Check sheet for the modelled part. Datum: model origin and axes. Units: mm. A direction names the side the tool comes from. Round coordinates to 2 decimals unless told otherwise and drop trailing zeros. Order: outer loops, then holes, each group sorted by start corner. A loop starts at its lowest first (then second) coordinate and runs counter-clockwise, first axis right, second up.
Q1. Set-up check for faces 1 (the cylindrical face through (17.15, 2.46, -19.99)), 2 (the flat face through (50, 3.48, -6.03)): record each of +Z, -Z, +X, -X, +Y, -Y from which the full face is reachable in a straight line by a thin tool's end or side.
Q2. Cross-section at D-D on x = 33. Record the cut outline in (y, z).
Q3. Depth check by flat-ended pin: P1, Ø5, axis at x = 5, z = 28, coming from the -Y side; P2, Ø12, axis at x = 39.31, z = -8.69, coming from the +Y side; P3, Ø2, axis at y = 1.5, z = 25.5, coming from the -X side; P4, Ø1, axis at x = -43, y = 3.5, coming from the -Z side. Enter the tip coordinate at first touch or a pass-through.
Q4. Cross-section at A-A on x = -5. Record the cut outline in (y, z), then the cut area to 3 significant figures.
Q5. Cross-section at C-C on y = 3.5. Give the number of separate pieces and of enclosed holes in the cut face, then the cut area to 3 significant figures.
Q6. Scan lines: probe 1 along X at (y, z) = (2.75, -28); probe 2 along Z at (x, y) = (17.5, 3.6); probe 3 along Z at (x, y) = (-8.5, 4.5). Record each from-to range of solid material in increasing order.
Q7. Cross-section at B-B on z = 28. Record the cut outline in (x, y).
from build123d import *

# Parameters (mm, degrees)
CROQUIS1_R              = 1.6
CROQUIS1_R_2            = 4.6875
SALIENTE_EXTRUIR1_DEPTH = 5
CORTAR_EXTRUIR1_START   = -3
CROQUIS2_R              = 3
CROQUIS2_R_2            = 1.6
CROQUIS2_R_3            = 4.6875
CORTAR_EXTRUIR1_DEPTH   = 3


with BuildPart() as part:
    # Croquis1 → Saliente-Extruir1 (new body)
    with BuildSketch(Plane(origin=(0, 0, 0), x_dir=(1, 0, 0), z_dir=(0, 1, 0))):
        with BuildLine():
            Line((-30, -33), (30, -33))
            ThreePointArc((30, -33), (47.67766953, -25.67766953), (55, -8))
            Line((55, -8), (55, 13))
            ThreePointArc((55, 13), (49.142135624, 27.142135624), (35, 33))
            Line((35, 33), (-35, 33))
            ThreePointArc((-35, 33), (-49.142135624, 27.142135624), (-55, 13))
            Line((-55, 13), (-55, -8))
            ThreePointArc((-55, -8), (-47.67766953, -25.67766953), (-30, -33))
        make_face()
        with Locations(Location((5, -28, 0), (0, 0, 270))):
            Circle(CROQUIS1_R, mode=Mode.SUBTRACT)
        with Locations(Location((20, 28, 0), (0, 0, 270))):
            Circle(CROQUIS1_R, mode=Mode.SUBTRACT)
        with Locations(Location((39.3125, 8.6875, 0), (0, 0, 270))):
            Circle(CROQUIS1_R_2, mode=Mode.SUBTRACT)
        with Locations(Location((-5, -28, 0), (0, 0, 90))):
            Circle(CROQUIS1_R, mode=Mode.SUBTRACT)
        with Locations(Location((-39.3125, 8.6875, 0), (0, 0, 90))):
            Circle(CROQUIS1_R_2, mode=Mode.SUBTRACT)
        with Locations(Location((-20, 28, 0), (0, 0, 90))):
            Circle(CROQUIS1_R, mode=Mode.SUBTRACT)
        with BuildLine():
            Line((-10, -23), (10, -23))
            ThreePointArc((10, -23), (17.071067812, -20.071067812), (20, -13))
            Line((20, -13), (20, 13))
            ThreePointArc((20, 13), (17.071067812, 20.071067812), (10, 23))
            Line((10, 23), (-10, 23))
            ThreePointArc((-10, 23), (-17.071067812, 20.071067812), (-20, 13))
            Line((-20, 13), (-20, -13))
            ThreePointArc((-20, -13), (-17.071067812, -20.071067812), (-10, -23))
        make_face(mode=Mode.SUBTRACT)
    extrude(amount=SALIENTE_EXTRUIR1_DEPTH)

    # Croquis2 → Cortar-Extruir1 (cut)
    # profile 1 of 6: a face of its own
    with BuildSketch(Plane(origin=(0, 5, 0), x_dir=(1, 0, 0), z_dir=(0, 1, 0)).offset(CORTAR_EXTRUIR1_START)):
        with Locations(Location((20, 28, 0), (0, 0, 270))):
            Circle(CROQUIS2_R)
        with Locations(Location((20, 28, 0), (0, 0, 270))):
            Circle(CROQUIS2_R_2, mode=Mode.SUBTRACT)
    # profile 2 of 6: a face of its own
    with BuildSketch(Plane(origin=(0, 5, 0), x_dir=(1, 0, 0), z_dir=(0, 1, 0)).offset(CORTAR_EXTRUIR1_START)):
        with Locations(Location((5, -28, 0), (0, 0, 270))):
            Circle(CROQUIS2_R)
        with Locations(Location((5, -28, 0), (0, 0, 270))):
            Circle(CROQUIS2_R_2, mode=Mode.SUBTRACT)
    # profile 3 of 6: a face of its own
    with BuildSketch(Plane(origin=(0, 5, 0), x_dir=(1, 0, 0), z_dir=(0, 1, 0)).offset(CORTAR_EXTRUIR1_START)):
        with Locations(Location((-5, -28, 0), (0, 0, 90))):
            Circle(CROQUIS2_R)
    # profile 4 of 6: a face of its own
    with BuildSketch(Plane(origin=(0, 5, 0), x_dir=(1, 0, 0), z_dir=(0, 1, 0)).offset(CORTAR_EXTRUIR1_START)):
        with Locations(Location((-20, 28, 0), (0, 0, 90))):
            Circle(CROQUIS2_R)
    # profile 5 of 6: a face of its own
    with BuildSketch(Plane(origin=(0, 5, 0), x_dir=(1, 0, 0), z_dir=(0, 1, 0)).offset(CORTAR_EXTRUIR1_START)):
        with BuildLine():
            Line((35.705717307, 16.009871883), (36.849149414, 22.614001921))
            ThreePointArc((36.849149414, 22.614001921), (39.3125, 24.6875), (41.775850586, 22.614001921))
            Line((41.775850586, 22.614001921), (42.919282693, 16.009871883))
            ThreePointArc((42.919282693, 16.009871883), (43.259020857, 15.523074638), (43.85046872, 15.472251379))
            Line((43.85046872, 15.472251379), (50.141529157, 17.784075147))
            ThreePointArc((50.141529157, 17.784075147), (53.168906461, 16.6875), (52.604879743, 13.517426775))
            Line((52.604879743, 13.517426775), (47.457251413, 9.225120503))
            ThreePointArc((47.457251413, 9.225120503), (47.205541715, 8.6875), (47.457251413, 8.149879497))
            Line((47.457251413, 8.149879497), (52.604879743, 3.857573225))
            ThreePointArc((52.604879743, 3.857573225), (53.168906461, 0.6875), (50.141529157, -0.409075147))
            Line((50.141529157, -0.409075147), (43.85046872, 1.902748621))
            ThreePointArc((43.85046872, 1.902748621), (43.259020857, 1.851925362), (42.919282693, 1.365128117))
            Line((42.919282693, 1.365128117), (41.775850586, -5.239001921))
            ThreePointArc((41.775850586, -5.239001921), (39.3125, -7.3125), (36.849149414, -5.239001921))
            Line((36.849149414, -5.239001921), (35.705717307, 1.365128117))
            ThreePointArc((35.705717307, 1.365128117), (35.365979143, 1.851925362), (34.77453128, 1.902748621))
            Line((34.77453128, 1.902748621), (28.483470843, -0.409075147))
            ThreePointArc((28.483470843, -0.409075147), (25.456093539, 0.6875), (26.020120257, 3.857573225))
            Line((26.020120257, 3.857573225), (31.167748587, 8.149879497))
            ThreePointArc((31.167748587, 8.149879497), (31.419458285, 8.6875), (31.167748587, 9.225120503))
            Line((31.167748587, 9.225120503), (26.020120257, 13.517426775))
            ThreePointArc((26.020120257, 13.517426775), (25.456093539, 16.6875), (28.483470843, 17.784075147))
            Line((28.483470843, 17.784075147), (34.77453128, 15.472251379))
            ThreePointArc((34.77453128, 15.472251379), (35.365979143, 15.523074638), (35.705717307, 16.009871883))
        make_face()
        with Locations(Location((39.3125, 8.6875, 0), (0, 0, 270))):
            Circle(CROQUIS2_R_3, mode=Mode.SUBTRACT)
    # profile 6 of 6: a face of its own
    with BuildSketch(Plane(origin=(0, 5, 0), x_dir=(1, 0, 0), z_dir=(0, 1, 0)).offset(CORTAR_EXTRUIR1_START)):
        with BuildLine():
            Line((-34.77453128, 15.472251379), (-28.483470843, 17.784075147))
            ThreePointArc((-28.483470843, 17.784075147), (-25.456093539, 16.6875), (-26.020120257, 13.517426775))
            Line((-26.020120257, 13.517426775), (-31.167748587, 9.225120503))
            ThreePointArc((-31.167748587, 9.225120503), (-31.419458285, 8.6875), (-31.167748587, 8.149879497))
            Line((-31.167748587, 8.149879497), (-26.020120257, 3.857573225))
            ThreePointArc((-26.020120257, 3.857573225), (-25.456093539, 0.6875), (-28.483470843, -0.409075147))
            Line((-28.483470843, -0.409075147), (-34.77453128, 1.902748621))
            ThreePointArc((-34.77453128, 1.902748621), (-35.365979143, 1.851925362), (-35.705717307, 1.365128117))
            Line((-35.705717307, 1.365128117), (-36.849149414, -5.239001921))
            ThreePointArc((-36.849149414, -5.239001921), (-39.3125, -7.3125), (-41.775850586, -5.239001921))
            Line((-41.775850586, -5.239001921), (-42.919282693, 1.365128117))
            ThreePointArc((-42.919282693, 1.365128117), (-43.259020857, 1.851925362), (-43.85046872, 1.902748621))
            Line((-43.85046872, 1.902748621), (-50.141529157, -0.409075147))
            ThreePointArc((-50.141529157, -0.409075147), (-53.168906461, 0.6875), (-52.604879743, 3.857573225))
            Line((-52.604879743, 3.857573225), (-47.457251413, 8.149879497))
            ThreePointArc((-47.457251413, 8.149879497), (-47.205541715, 8.6875), (-47.457251413, 9.225120503))
            Line((-47.457251413, 9.225120503), (-52.604879743, 13.517426775))
            ThreePointArc((-52.604879743, 13.517426775), (-53.168906461, 16.6875), (-50.141529157, 17.784075147))
            Line((-50.141529157, 17.784075147), (-43.85046872, 15.472251379))
            ThreePointArc((-43.85046872, 15.472251379), (-43.259020857, 15.523074638), (-42.919282693, 16.009871883))
            Line((-42.919282693, 16.009871883), (-41.775850586, 22.614001921))
            ThreePointArc((-41.775850586, 22.614001921), (-39.3125, 24.6875), (-36.849149414, 22.614001921))
            Line((-36.849149414, 22.614001921), (-35.705717307, 16.009871883))
            ThreePointArc((-35.705717307, 16.009871883), (-35.365979143, 15.523074638), (-34.77453128, 15.472251379))
        make_face()
    extrude(amount=CORTAR_EXTRUIR1_DEPTH, mode=Mode.SUBTRACT)


solid = part.part
Results found:
1. face 1: +Y, -Y
1. face 2: +Y
2. outline: (0, -33) - (5, -33) - (5, -16.12) - (2, -16.12) - (2, -1.25) - (5, -1.25) - (5, 32.82) - (0, 32.82) - close
3. P1: stops at y = 0
3. P2: stops at y = 2
3. P3: stops at x = -48.78
3. P4: stops at z = -31.54
4. outline: (0, -33) - (5, -33) - (5, -23) - (0, -23) - close; (0, 23) - (5, 23) - (5, 25) - (2, 25) - (2, 26.4) - (0, 26.4) - close; (0, 29.6) - (2, 29.6) - (2, 31) - (5, 31) - (5, 33) - (0, 33) - close
4. area: 75.6 mm2
5. separate pieces: 1
5. enclosed holes: 7
5. area: 4,010 mm2
6. probe 1: x = -48.23 to -23, -17 to 17, 23 to 48.23
6. probe 2: z = -33 to -29.66, -26.34 to -19.61, 19.61 to 33
6. probe 3: z = -33 to -23, 23 to 33
7. outline: (-45, 0) - (-6.6, 0) - (-6.6, 2) - (-8, 2) - (-8, 5) - (-45, 5) - close; (-3.4, 0) - (3.4, 0) - (3.4, 2) - (2, 2) - (2, 5) - (-2, 5) - (-2, 2) - (-3.4, 2) - close; (6.6, 0) - (45, 0) - (45, 5) - (8, 5) - (8, 2) - (6.6, 2) - close
